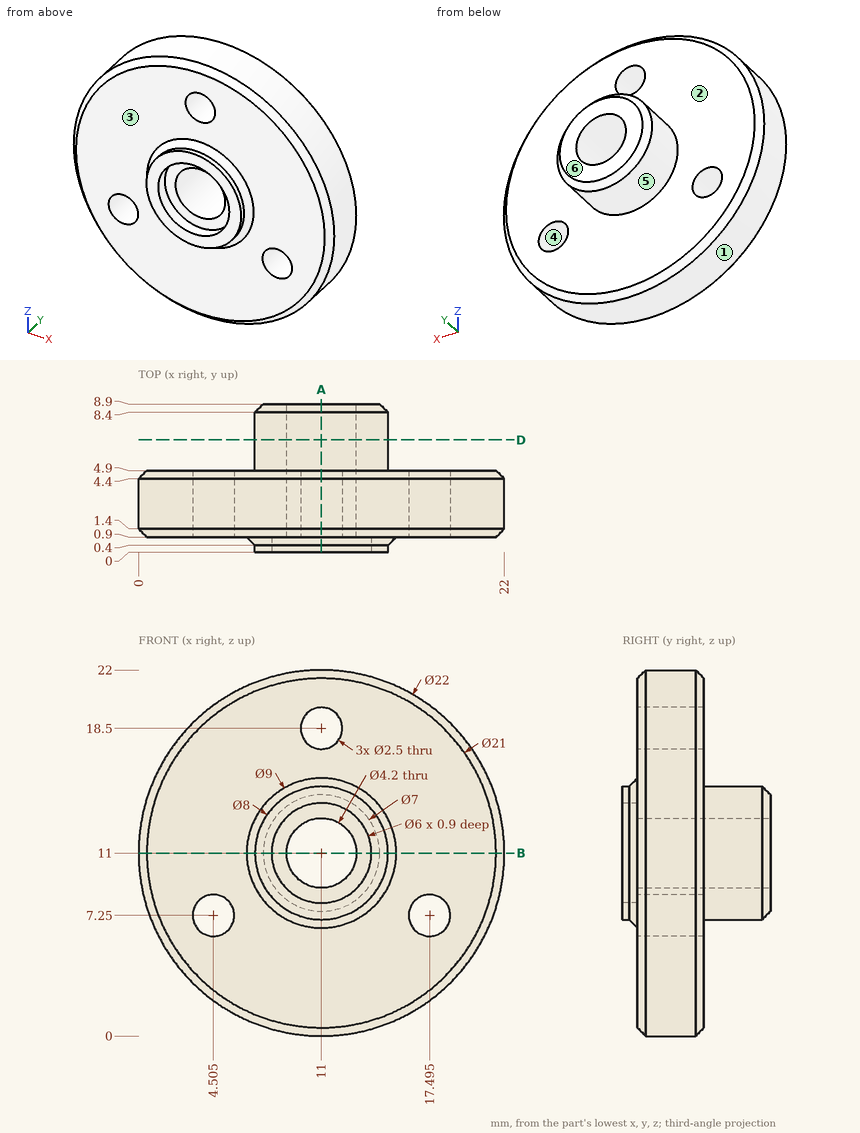
Answer from the drawing. Dimensions are ordinates in mm from the lowest x, y and z of the part. A direction names the side the tool comes from. Give positions to 0.01 mm unless a question says otherwise; leave off trailing zeros. Loops run counter-clockwise (first coordinate to the right, second up) from the corner with the lowest first, then second, coordinate; pieces in that order, holes last. Notation, with made-up numbers: (-4.75, 87) - (4.25, 87) arc R29 ccw to (4.25, 119) - close; hole circle Ø2 at (89.25, -27). An arc over 180 degrees is marked (long way). Answer as CSV lines item,"result". Start each with the question number.
Item 1: Find the intervals of material crossed by line 1 (Z direction, x = 11, y = 0.25); line 2 (Z direction, x = 10.5, y = 4.5) (1 decimal); line 3 (Y direction, x = 9.75, z = 1.5), in increasing order. Write a range as from..to.
Item 2: For the marked faces 1, 2 and 3, determine the directions among +Z, -Z, +X, -X, +Y, -Y from which every point of the face is accessible in a straight line to the end or side of a thin tool.
Item 3: The mould has two halves that part along Z. Classify the marked faces 4, 5 and 6: +Z half, -Z half, draft (parallel to the pull), parting line (faces both ways), or undercut.
Item 4: A cutting plane is placed at D-D on y = 6.75. Determine the outline of the cut face in (x, z), then the cut area to 3 significant figures.
Item 5: A cutting plane is placed at A-A on x = 11. Count the separate pieces of the cut face and the enclosed holes in it, then the cut area to 3 significant figures.
Item 6: Each of these flat-tipped pins is pushed along its axis until it touches: pin 1 (3 mm diameter, centred on x = 12.5, z = 3, fed in from -Y); pin 2 (2 mm diameter, centred on y = 2, z = 7.5, fed in from -X); pin 3 (6.5 mm diameter, centred on x = 12, z = 9, fed in from -Y); pin 4 (1 mm diameter, centred on y = 2.5, z = 19.5, fed in from -X). Where does it stop, or does it pass through?
Item 7: A cutting plane is placed at B-B on z = 11. Determine the outline of the cut face in (x, y), then the cut area to 3 significant figures.
Found:
1,line 1,"z = 7..8, 14..15"
1,line 2,"z = 0.1..9, 13..17.4, 19.6..21.9"
1,line 3,"y = 0.9..4.9"
2,face 1,"+Y, -Y"
2,face 2,"+Y"
2,face 3,"-Y"
3,face 4,"undercut"
3,face 5,"parting line"
3,face 6,"draft"
4,outline,"circle Ø8 at (11, 11); hole circle Ø4.2 at (11, 11)"
4,area,"36.4 mm^2"
5,separate pieces,"3"
5,enclosed holes,"0"
5,area,"77.7 mm^2"
6,pin 1,"stops at y = 0.9"
6,pin 2,"stops at x = 0.29"
6,pin 3,"stops at y = 0"
6,pin 4,"stops at x = 3.45"
7,outline,"(0, 1.4) - (0.5, 0.9) - (6.5, 0.9) - (7, 0.4) - (7, 0) - (8, 0) - (8, 0.9) - (8.9, 0.9) - (8.9, 8.9) - (7.5, 8.9) - (7, 8.4) - (7, 4.9) - (0.5, 4.9) - (0, 4.4) - close; (13.1, 0.9) - (14, 0.9) - (14, 0) - (15, 0) - (15, 0.4) - (15.5, 0.9) - (21.5, 0.9) - (22, 1.4) - (22, 4.4) - (21.5, 4.9) - (15, 4.9) - (15, 8.4) - (14.5, 8.9) - (13.1, 8.9) - close"
7,area,"87.7 mm^2"
